For this review, use the dimensioned drawing (mm, ordinates from the lowest corner) and the shaded views. A direction names the side the tool comes from. Coordinates: 2 decimals unless noted, no trailing zeros. Order: outer loops, then holes, each group sorted by start corner. A loop starts at its lowest first (then second) coordinate and runs counter-clockwise, first axis right, second up. Notation, with made-up numbers: M 28.5,63.5 L 37.5,63.5 A33 ccw 37.5,95.5 Z; hole C 29,-37.5 d4. An arc over 180 degrees is marked long. Answer in a Markdown table with one row per item.
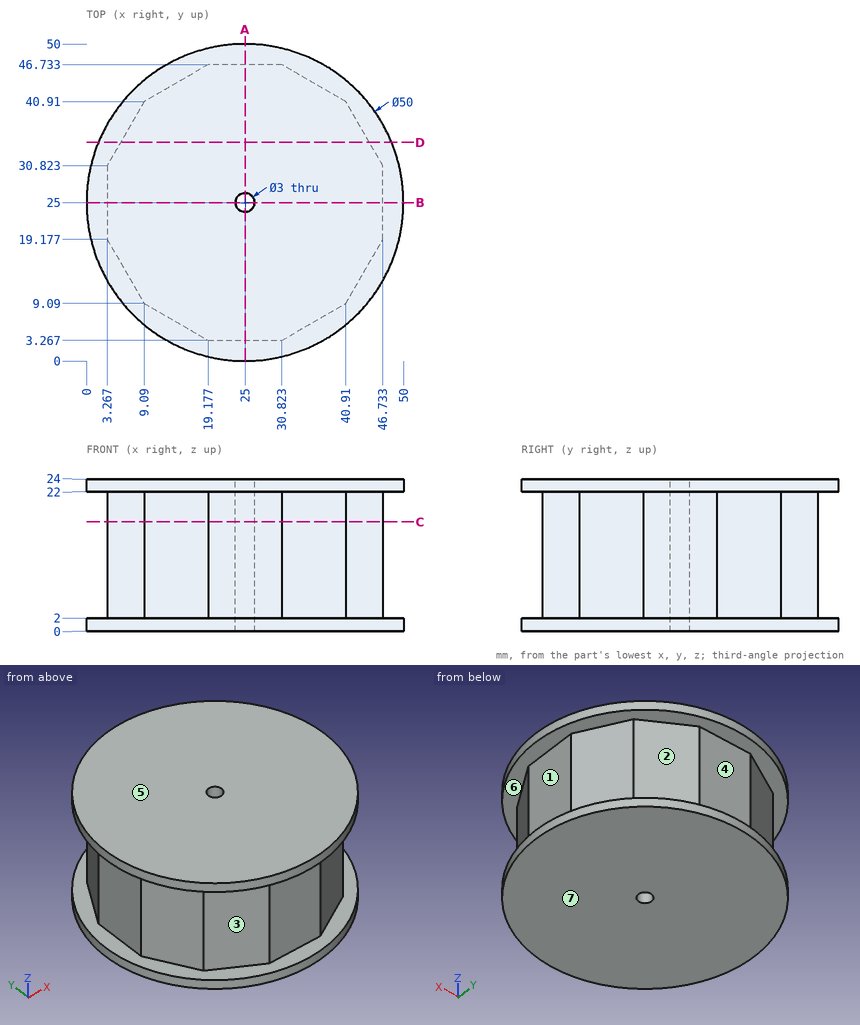
(1) Take a section at D-D (y = 34.5). Write out the cut boundary in (x, z) (1 decimal).
Report:
| item | result |
|---|---|
| outline | M 1.9,0 L 48.1,0 L 48.1,2 L 44.6,2 L 44.6,22 L 48.1,22 L 48.1,24 L 1.9,24 L 1.9,22 L 5.4,22 L 5.4,2 L 1.9,2 Z |
(2) Take a section at A-A (x = 25). Write out the cut boundary in (y, z), then the cut area to 3 significant figures.
Report:
| item | result |
|---|---|
| outline | M 0,0 L 23.5,0 L 23.5,24 L 0,24 L 0,22 L 3.27,22 L 3.27,2 L 0,2 Z; M 26.5,0 L 50,0 L 50,2 L 46.73,2 L 46.73,22 L 50,22 L 50,24 L 26.5,24 Z |
| area | 997 mm^2 |
(3) The part is to be moulded in two halves that separate along Z. For the marked faces 5, 6 and 7, say which applies: +Z half, -Z half, draft (parallel to the pull), parting line (faces both ways), or undercut.
Report:
| item | result |
|---|---|
| face 5 | +Z half |
| face 6 | undercut |
| face 7 | -Z half |
(4) To check wall thickness, follow line 1 (Y direction, x = 25, z = 12); line 2 (Z direction, x = 4.5, y = 38.5). State the ranges of each line that lie inside material, in increasing order. Write a range as [from, to].
Report:
| item | result |
|---|---|
| line 1 | [3.27, 23.5], [26.5, 46.73] |
| line 2 | [0, 2], [22, 24] |
(5) Take a section at C-C (z = 17.25). Write out the cut boundary in (x, y), then the cut area to 3 significant figures.
Report:
| item | result |
|---|---|
| outline | M 3.27,19.18 L 9.09,9.09 L 19.18,3.27 L 30.82,3.27 L 40.91,9.09 L 46.73,19.18 L 46.73,30.82 L 40.91,40.91 L 30.82,46.73 L 19.18,46.73 L 9.09,40.91 L 3.27,30.82 Z; hole C 25,25 d3 |
| area | 1,510 mm^2 |
(6) Insertion check: P1, Ø10, axis at y = 11.5, z = 8.5, coming from the +X side; P2, Ø4, axis at y = 5, z = 12, coming from the -X side; P3, Ø6, axis at x = 27.5, z = 8.5, coming from the +Y side. Each pin has a flat end and moves straight along its axis. Give the tip position at first contact, or say it passes through.
Report:
| item | result |
|---|---|
| P1 | x = 45.19 |
| P2 | x = 12.71 |
| P3 | y = 46.73 |
(7) Machinability: for the marked faces 1, 2, 3 and 4, which of the approach directions +Z, -Z, +X, -X, +Y, -Y give a long, thin tool a straight path to every point of the face, cutting with its end or side? Answer none if there is none.
Report:
| item | result |
|---|---|
| face 1 | +X, +Y, -Y |
| face 2 | +X, +Y |
| face 3 | -X, -Y |
| face 4 | +X, -X, +Y |
